Check sheet for the modelled part. Datum: model origin and axes. Units: mm. A direction names the side the tool comes from. Round coordinates to 2 decimals unless told otherwise and drop trailing zeros. Write each loop counter-clockwise with the first axis right and the second up, starting at its lowest first coordinate (ties: lowest second). Pieces come first, ordered by that corner, then holes. Notation, with made-up numbers: (-9.5, 27.5) - (2.5, 27.5) arc R34 ccw to (2.5, 57.5) - close; hole circle Ø7 at (48, 3). An arc over 180 degrees is marked (long way). Use one line per item in the form item = value. Start each with the question number.
1) Section check C-C (x = -6). Record the boundary of the cut face in (y, z), then the cut area to 3 significant figures.
2) Section check A-A (y = 0). Record the boundary of the cut face in (x, z).
3) Scan lines: probe 1 along X at (y, z) = (-3.5, 4); probe 2 along Z at (x, y) = (-20.5, -3.25); probe 3 along Z at (x, y) = (9.5, 3.75). Record each from-to range of solid material in increasing order.
4) Set-up check for faces 1 (the face through (-30, 0, 0)), 2 (the face through (0, 0, -5)): record each of +Z, -Z, +X, -X, +Y, -Y from which the full face is reachable in a straight line by a thin tool's end or side.
5) Gauge pin test, flat ends, axial feed: P1, Ø5, axis at x = 4, y = 2.5, coming from the +Z side; P2, Ø5, axis at x = -18.5, z = -5, coming from the -Y side; P3, Ø5, axis at x = 0.5, y = 4, coming from the -Z side. Record the tip position at first contact, or that the pin passes through.
6) Section check D-D (z = 5.25). Record the boundary of the cut face in (x, y).
from build123d import *

# Parameters (mm, degrees)
SKETCH_1_R      = 8
EXTRUDE_1_DEPTH = 30
SKETCH_2_R      = 4.75
EXTRUDE_2_DEPTH = 25
CHAMFER_1_SIZE  = 3


with BuildPart() as part:
    # Эскиз1 → Бобышка-Вытянуть1 (new body)
    with BuildSketch(Plane(origin=(0, 0, 0), x_dir=(0, 0, -1), z_dir=(1, 0, 0))):
        Circle(SKETCH_1_R)
    extrude(amount=-EXTRUDE_1_DEPTH)

    # Эскиз2 → Бобышка-Вытянуть2 (add)
    with BuildSketch(Plane(origin=(0, 0, 0), x_dir=(0, 0, -1), z_dir=(1, 0, 0))):
        Circle(SKETCH_2_R)
    extrude(amount=EXTRUDE_2_DEPTH)

    # Фаска1
    chamfer_1_edges = [part.edges().sort_by_distance(p)[0] for p in [
        (25, 0, 4.75),
    ]]
    chamfer(chamfer_1_edges, length=CHAMFER_1_SIZE)


solid = part.part
Results are:
q1.outline = circle Ø16 at (0, 0)
q1.area = 201 mm²
q2.outline = (-30, -8) - (0, -8) - (0, -4.75) - (22, -4.75) - (25, -1.75) - (25, 1.75) - (22, 4.75) - (0, 4.75) - (0, 8) - (-30, 8) - close
q3.probe_1 = -30 to 0
q3.probe_2 = -7.31 to 7.31
q3.probe_3 = -2.92 to 2.92
q4.face_1 = +Z, -Z, -X, +Y, -Y
q4.face_2 = +X
q5.P1 = 4.75
q5.P2 = -7.6
q5.P3 = -7.85
q6.outline = (-30, -6.04) - (0, -6.04) - (0, 6.04) - (-30, 6.04) - close
